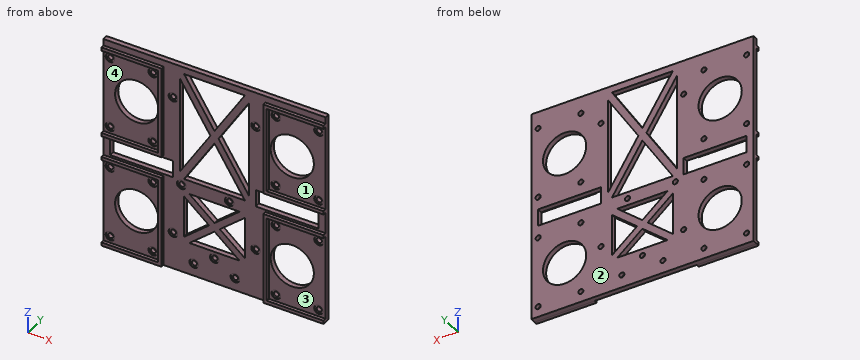
from build123d import *

# Parameters (mm, degrees)
SKETCH1_W                 = 130
SKETCH1_H                 = 125
BOSS_EXTRUDE1_DEPTH       = 5
SKETCH2_R                 = 1.5
SKETCH2_R_2               = 12.65
CUT_EXTRUDE1_DEPTH        = 10
SKETCH4_R                 = 1.5
CUT_EXTRUDE3_DEPTH        = 10
BOSS_EXTRUDE2_DEPTH       = 2
MIRROR7_COPY_1_SKETCH_R   = 1.5
MIRROR7_COPY_1_SKETCH_R_2 = 12.65
MIRROR7_COPY_1_DEPTH      = 10
MIRROR7_COPY_2_DEPTH      = 2
SKETCH10_R                = 1.5
CUT_EXTRUDE8_DEPTH        = 91.311959341
SKETCH11_R                = 2.65
CUT_EXTRUDE9_DEPTH        = 0.5
CUT_EXTRUDE10_DEPTH       = 91.444734507
CUT_EXTRUDE11_DEPTH       = 91.444734507
CUT_EXTRUDE12_DEPTH       = 91.444734507
SKETCH15_W                = 130
SKETCH15_H                = 125
SKETCH15_W_2              = 5
SKETCH15_H_2              = 5
CUT_EXTRUDE14_DEPTH       = 2
CUT_EXTRUDE15_START       = -8
SKETCH17_W                = 137.629855092
SKETCH17_H                = 131.076052468
CUT_EXTRUDE15_DEPTH       = 2


with BuildPart() as part:
    # Sketch1 → Boss-Extrude1 (new body)
    with BuildSketch(Plane(origin=(0, 0, 0), x_dir=(1, 0, 0), z_dir=(0, 1, 0))):
        Rectangle(SKETCH1_W, SKETCH1_H)
    extrude(amount=BOSS_EXTRUDE1_DEPTH)

    # Sketch2 → Cut-Extrude1 (cut)
    with BuildSketch(Plane(origin=(0, 5, 0), x_dir=(1, 0, 0), z_dir=(0, 1, 0))):
        with Locations(Location((-61, -52.5, 0), (0, 0, 270))):
            Circle(SKETCH2_R)
        with Locations(Location((-36, -52.5, 0), (0, 0, 270))):
            Circle(SKETCH2_R)
        with Locations(Location((-36, -10.5, 0), (0, 0, 270))):
            Circle(SKETCH2_R)
        with Locations(Location((-61, -10.5, 0), (0, 0, 270))):
            Circle(SKETCH2_R)
        with Locations(Location((-45.5, -31.5, 0), (0, 0, 270))):
            Circle(SKETCH2_R_2)
    cut_extrude1 = extrude(amount=-CUT_EXTRUDE1_DEPTH, mode=Mode.SUBTRACT)

    # Mirror3: Cut-Extrude1 across plane
    add(cut_extrude1.mirror(Plane.ZY), mode=Mode.SUBTRACT)

    # Sketch4 → Cut-Extrude3 (cut)
    with BuildSketch(Plane(origin=(0, 5, 0), x_dir=(1, 0, 0), z_dir=(0, 1, 0))):
        with Locations(Location((0, 47.5, 0), (0, 0, 270))):
            Circle(SKETCH4_R)
        with Locations(Location((12.049810205, 55, 0), (0, 0, 270))):
            Circle(SKETCH4_R)
        with Locations(Location((-12.049810205, 55, 0), (0, 0, 270))):
            Circle(SKETCH4_R)
    extrude(amount=-CUT_EXTRUDE3_DEPTH, mode=Mode.SUBTRACT)

    # Sketch5 → Boss-Extrude2 (add)
    with BuildSketch(Plane.XZ):
        Polygon((-65, 58.6), (-65, 56.6), (-31.8, 56.6), (-31.8, 6.4), (-65, 6.4), (-65, 4.4), (-29.8, 4.4), (-29.8, 58.6), align=None)
    boss_extrude2 = extrude(amount=BOSS_EXTRUDE2_DEPTH)

    # Mirror5: Boss-Extrude2 across plane
    add(boss_extrude2.mirror(Plane.ZY))

    # Mirror7: Cut-Extrude1, Boss-Extrude2 across plane
    add(cut_extrude1.mirror(Plane.XY.offset(-1.9)), mode=Mode.SUBTRACT)
    add(boss_extrude2.mirror(Plane.XY.offset(-1.9)))

    # Mirror7 copy 1 sketch → Mirror7 copy 1 (cut)
    with BuildSketch(Plane(origin=(0, 5, -3.8), x_dir=(-1, 0, 0), z_dir=(0, 1, 0))):
        with Locations(Location((-61, -52.5, 0), (0, 0, 270))):
            Circle(MIRROR7_COPY_1_SKETCH_R)
        with Locations(Location((-36, -52.5, 0), (0, 0, 270))):
            Circle(MIRROR7_COPY_1_SKETCH_R)
        with Locations(Location((-36, -10.5, 0), (0, 0, 270))):
            Circle(MIRROR7_COPY_1_SKETCH_R)
        with Locations(Location((-61, -10.5, 0), (0, 0, 270))):
            Circle(MIRROR7_COPY_1_SKETCH_R)
        with Locations(Location((-45.5, -31.5, 0), (0, 0, 270))):
            Circle(MIRROR7_COPY_1_SKETCH_R_2)
    extrude(amount=-MIRROR7_COPY_1_DEPTH, mode=Mode.SUBTRACT)

    # Mirror7 copy 2 sketch → Mirror7 copy 2 (add)
    with BuildSketch(Plane(origin=(0, 0, -3.8), x_dir=(-1, 0, 0), z_dir=(0, -1, 0))):
        Polygon((-65, 58.6), (-65, 56.6), (-31.8, 56.6), (-31.8, 6.4), (-65, 6.4), (-65, 4.4), (-29.8, 4.4), (-29.8, 58.6), align=None)
    extrude(amount=MIRROR7_COPY_2_DEPTH)

    # Sketch10 → Cut-Extrude8 (cut, through all)
    with BuildSketch(Plane(origin=(0, 0, 0), x_dir=(-1, 0, 0), z_dir=(0, -1, 0))):
        with Locations(Location((-24.17, -42.03, 0), (0, 0, 90))):
            Circle(SKETCH10_R)
        with Locations(Location((24.17, -42.03, 0), (0, 0, 90))):
            Circle(SKETCH10_R)
        with Locations(Location((-8.73, 9.6, 0), (0, 0, 90))):
            Circle(SKETCH10_R)
        with Locations(Location((19.29, 9.6, 0), (0, 0, 90))):
            Circle(SKETCH10_R)
        with Locations(Location((-24.17, 33.11, 0), (0, 0, 90))):
            Circle(SKETCH10_R)
        with Locations(Location((24.17, 40.6, 0), (0, 0, 90))):
            Circle(SKETCH10_R)
    extrude(amount=-CUT_EXTRUDE8_DEPTH, mode=Mode.SUBTRACT)

    # Sketch11 → Cut-Extrude9 (cut)
    with BuildSketch(Plane.XZ):
        with Locations(Location((-12.049810205, -55, 0), (0, 0, 270))):
            Circle(SKETCH11_R)
        with Locations(Location((0, -47.5, 0), (0, 0, 270))):
            Circle(SKETCH11_R)
        with Locations(Location((12.049810205, -55, 0), (0, 0, 270))):
            Circle(SKETCH11_R)
        with Locations(Location((-24.17, -40.6, 0), (0, 0, 270))):
            Circle(SKETCH11_R)
        with Locations(Location((24.17, -33.11, 0), (0, 0, 270))):
            Circle(SKETCH11_R)
        with Locations(Location((8.73, -9.6, 0), (0, 0, 270))):
            Circle(SKETCH11_R)
        with Locations(Location((-19.29, -9.6, 0), (0, 0, 270))):
            Circle(SKETCH11_R)
        with Locations(Location((-24.17, 42.03, 0), (0, 0, 270))):
            Circle(SKETCH11_R)
        with Locations(Location((24.17, 42.03, 0), (0, 0, 270))):
            Circle(SKETCH11_R)
        with Locations(Location((-61, -14.3, 0), (0, 0, 270))):
            Circle(SKETCH11_R)
        with Locations(Location((-36, -14.3, 0), (0, 0, 270))):
            Circle(SKETCH11_R)
        with Locations(Location((-61, -56.3, 0), (0, 0, 270))):
            Circle(SKETCH11_R)
        with Locations(Location((-36, -56.3, 0), (0, 0, 270))):
            Circle(SKETCH11_R)
        with Locations(Location((36, -56.3, 0), (0, 0, 270))):
            Circle(SKETCH11_R)
        with Locations(Location((61, -56.3, 0), (0, 0, 270))):
            Circle(SKETCH11_R)
        with Locations(Location((36, -14.3, 0), (0, 0, 270))):
            Circle(SKETCH11_R)
        with Locations(Location((61, -14.3, 0), (0, 0, 270))):
            Circle(SKETCH11_R)
        with Locations(Location((36, 10.5, 0), (0, 0, 270))):
            Circle(SKETCH11_R)
        with Locations(Location((61, 10.5, 0), (0, 0, 270))):
            Circle(SKETCH11_R)
        with Locations(Location((61, 52.5, 0), (0, 0, 270))):
            Circle(SKETCH11_R)
        with Locations(Location((36, 52.5, 0), (0, 0, 270))):
            Circle(SKETCH11_R)
        with Locations(Location((-36, 52.5, 0), (0, 0, 270))):
            Circle(SKETCH11_R)
        with Locations(Location((-36, 10.5, 0), (0, 0, 270))):
            Circle(SKETCH11_R)
        with Locations(Location((-61, 10.5, 0), (0, 0, 270))):
            Circle(SKETCH11_R)
        with Locations(Location((-61, 52.5, 0), (0, 0, 270))):
            Circle(SKETCH11_R)
    extrude(amount=-CUT_EXTRUDE9_DEPTH, mode=Mode.SUBTRACT)

    # Sketch12 → Cut-Extrude10 (cut, through all)
    with BuildSketch(Plane(origin=(0, 5, 0), x_dir=(1, 0, 0), z_dir=(0, 1, 0))):
        Polygon((-2.363095604, -26.45), (-20.17, 1.845056316), (-20.17, -54.745056316), align=None)
        Polygon((17.806904396, 5.6), (-17.806904396, 5.6), (0, -22.695056316), align=None)
        Polygon((20.17, -54.745056316), (20.17, 1.845056316), (2.363095604, -26.45), align=None)
        Polygon((0, -30.204943684), (-17.806904396, -58.5), (17.806904396, -58.5), align=None)
    extrude(amount=-CUT_EXTRUDE10_DEPTH, mode=Mode.SUBTRACT)

    # Sketch13 → Cut-Extrude11 (cut, through all)
    with BuildSketch(Plane(origin=(0, 5, 0), x_dir=(1, 0, 0), z_dir=(0, 1, 0))):
        Polygon((-61, 1.9), (-61, -3.1), (-24.17, -3.1), (-24.17, 6.9), (-61, 6.9), align=None)
    cut_extrude11 = extrude(amount=-CUT_EXTRUDE11_DEPTH, mode=Mode.SUBTRACT)

    # Mirror9: Cut-Extrude11 across plane
    add(cut_extrude11.mirror(Plane.ZY), mode=Mode.SUBTRACT)

    # Sketch14 → Cut-Extrude12 (cut, through all)
    with BuildSketch(Plane(origin=(0, 5, 0), x_dir=(1, 0, 0), z_dir=(0, 1, 0))):
        Polygon((-3.110442245, 28.55), (-17.806904396, 40.888590935), (-17.806904396, 16.211409065), align=None)
        Polygon((14.696462151, 43.5), (-14.696462151, 43.5), (0, 31.161409065), align=None)
        Polygon((17.806904396, 16.211409065), (17.806904396, 40.888590935), (3.110442245, 28.55), align=None)
        Polygon((0, 25.938590935), (-14.696462151, 13.6), (14.696462151, 13.6), align=None)
    extrude(amount=-CUT_EXTRUDE12_DEPTH, mode=Mode.SUBTRACT)

    # Sketch15 → Cut-Extrude14 (cut)
    with BuildSketch(Plane(origin=(0, 5, 0), x_dir=(1, 0, 0), z_dir=(0, 1, 0))):
        Rectangle(SKETCH15_W, SKETCH15_H)
        with Locations((-61, 56.3)):
            Rectangle(SKETCH15_W_2, SKETCH15_H_2, mode=Mode.SUBTRACT)
        with Locations((-36, 56.3)):
            Rectangle(SKETCH15_W_2, SKETCH15_H_2, mode=Mode.SUBTRACT)
        with Locations((-12.049810205, 55)):
            Rectangle(SKETCH15_W_2, SKETCH15_H_2, mode=Mode.SUBTRACT)
        with Locations((0, 47.5)):
            Rectangle(SKETCH15_W_2, SKETCH15_H_2, mode=Mode.SUBTRACT)
        with Locations((12.049810205, 55)):
            Rectangle(SKETCH15_W_2, SKETCH15_H_2, mode=Mode.SUBTRACT)
        with Locations((36, 56.3)):
            Rectangle(SKETCH15_W_2, SKETCH15_H_2, mode=Mode.SUBTRACT)
        with Locations((61, 56.3)):
            Rectangle(SKETCH15_W_2, SKETCH15_H_2, mode=Mode.SUBTRACT)
        with Locations((36, 14.3)):
            Rectangle(SKETCH15_W_2, SKETCH15_H_2, mode=Mode.SUBTRACT)
        with Locations((61, 14.3)):
            Rectangle(SKETCH15_W_2, SKETCH15_H_2, mode=Mode.SUBTRACT)
        with Locations((24.17, 33.11)):
            Rectangle(SKETCH15_W_2, SKETCH15_H_2, mode=Mode.SUBTRACT)
        with Locations((36, -10.5)):
            Rectangle(SKETCH15_W_2, SKETCH15_H_2, mode=Mode.SUBTRACT)
        with Locations((61, -10.5)):
            Rectangle(SKETCH15_W_2, SKETCH15_H_2, mode=Mode.SUBTRACT)
        with Locations((24.17, -42.03)):
            Rectangle(SKETCH15_W_2, SKETCH15_H_2, mode=Mode.SUBTRACT)
        with Locations((36, -52.5)):
            Rectangle(SKETCH15_W_2, SKETCH15_H_2, mode=Mode.SUBTRACT)
        with Locations((61, -52.5)):
            Rectangle(SKETCH15_W_2, SKETCH15_H_2, mode=Mode.SUBTRACT)
        with Locations((-24.17, -42.03)):
            Rectangle(SKETCH15_W_2, SKETCH15_H_2, mode=Mode.SUBTRACT)
        with Locations((-36, -52.5)):
            Rectangle(SKETCH15_W_2, SKETCH15_H_2, mode=Mode.SUBTRACT)
        with Locations((-36, -10.5)):
            Rectangle(SKETCH15_W_2, SKETCH15_H_2, mode=Mode.SUBTRACT)
        with Locations((8.73, 9.6)):
            Rectangle(SKETCH15_W_2, SKETCH15_H_2, mode=Mode.SUBTRACT)
        with Locations((-19.29, 9.6)):
            Rectangle(SKETCH15_W_2, SKETCH15_H_2, mode=Mode.SUBTRACT)
        with Locations((-24.17, 40.6)):
            Rectangle(SKETCH15_W_2, SKETCH15_H_2, mode=Mode.SUBTRACT)
        with Locations((-61, 14.3)):
            Rectangle(SKETCH15_W_2, SKETCH15_H_2, mode=Mode.SUBTRACT)
        with Locations((-36, 14.3)):
            Rectangle(SKETCH15_W_2, SKETCH15_H_2, mode=Mode.SUBTRACT)
        with Locations((-61, -10.5)):
            Rectangle(SKETCH15_W_2, SKETCH15_H_2, mode=Mode.SUBTRACT)
        with Locations((-61, -52.5)):
            Rectangle(SKETCH15_W_2, SKETCH15_H_2, mode=Mode.SUBTRACT)
    extrude(amount=-CUT_EXTRUDE14_DEPTH, mode=Mode.SUBTRACT)

    # Sketch17 → Cut-Extrude15 (cut)
    with BuildSketch(Plane(origin=(0, 13, 0), x_dir=(1, 0, 0), z_dir=(0, 1, 0)).offset(CUT_EXTRUDE15_START)):
        with Locations((0.756207995, -1.260346658)):
            Rectangle(SKETCH17_W, SKETCH17_H)
    extrude(amount=-CUT_EXTRUDE15_DEPTH, mode=Mode.SUBTRACT)


solid = part.part
The model under review builds one solid part; all positions refer to its coordinate system, in mm. Face numbers are marked on the shaded views. A direction names the side the tool comes from. Round coordinates to 2 decimals unless told otherwise and drop trailing zeros. Write item = value, one per line. Start each with the question number.
Item 1: To check wall thickness, follow L1, parallel to X at y = -1.15, z = 13.5; L2, parallel to X at y = 1.9, z = 31.5; L3, parallel to X at y = 2.8, z = -36.5. State the ranges of each line that lie inside material, in increasing order.
Item 2: Take a section at A-A on y = -0.9. Count the separate pieces of the cut face and the enclosed holes in it, plus the area to 3 significant figures.
Item 3: Insertion check: pin 1 (1.5 mm diameter, centred on x = 13, z = -13.5, fed in from -Y); pin 2 (2.5 mm diameter, centred on x = 61.5, z = 10.5, fed in from -Y); pin 3 (0.6 mm diameter, centred on y = -0.5, z = -48, fed in from +X). Each pin has a flat end and moves straight along its axis. Give the tip position at first contact, or say it passes through.
Item 4: For the marked faces 3 and 4, list the 3-axis set-ups (+Z, -Z, +X, -X, +Y, -Y) from which the entire face can be reached by the end or side of a thin tool; tool diameter is ignored.
Item 5: Mouldability with a two-part tool opening along Z and no side actions: class the marked faces 1 and 2 as released by +Z, released by -Z, zero draft, split by the parting line, or undercut.
Result:
q1.L1 = -31.8 to -29.8, 29.8 to 31.8
q1.L2 = -65 to -58.15, -32.85 to -20.17, -5.54 to -0.82, 0.82 to 5.54, 20.17 to 32.85, 58.15 to 65
q1.L3 = -65 to -58.09, -32.91 to -17.81, -12.58 to -6.36, 6.36 to 12.58, 17.81 to 32.91, 58.09 to 65
q2.separate_pieces = 4
q2.enclosed_holes = 0
q2.area = 965 mm²
q3.pin_1 = 0
q3.pin_2 = 0.5
q3.pin_3 = 31.8
q4.face_3 = +X, -Y
q4.face_4 = -X, -Y
q5.face_1 = undercut
q5.face_2 = zero draft
